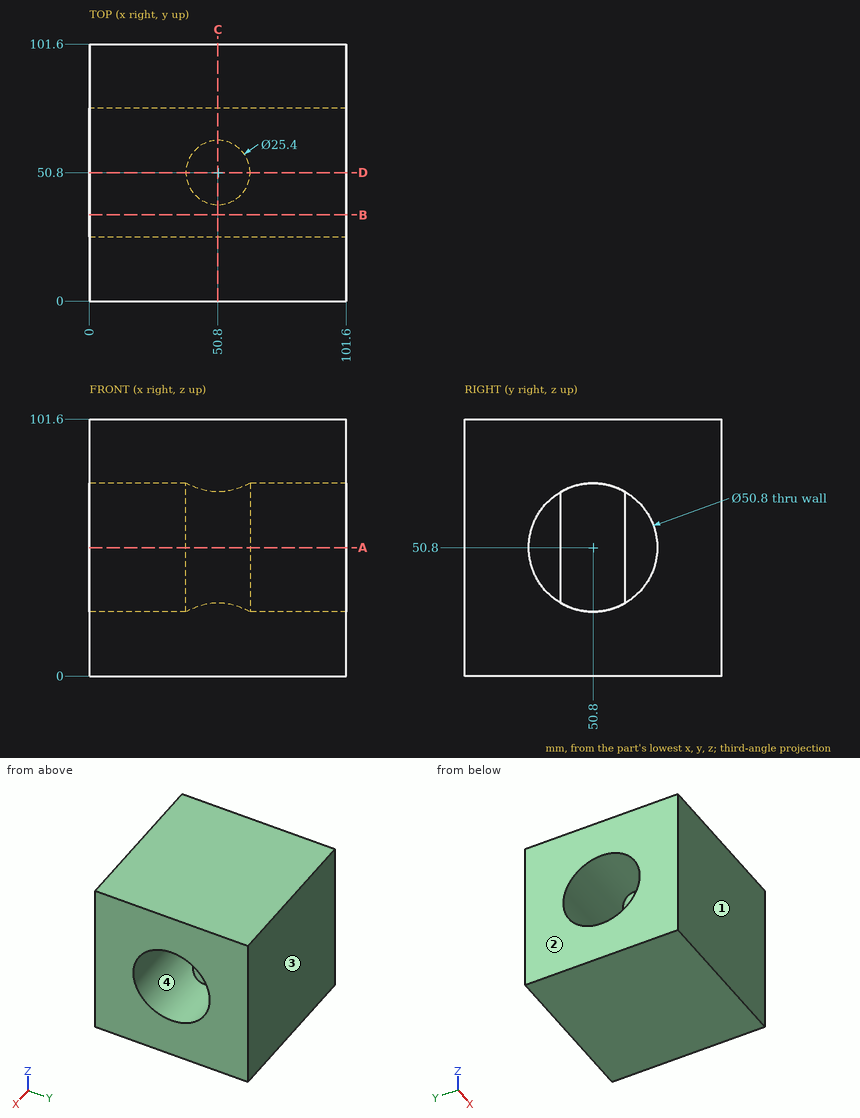
Input: dimensioned drawing with shaded views. Units: mm. Origin: part minimum x, y, z. Round coordinates to 2 decimals unless told otherwise and drop trailing zeros. Write each loop counter-clockwise with the first axis right and the second up, starting at its lowest first coordinate (ties: lowest second). Pieces come first, ordered by that corner, then holes. Notation, with made-up numbers: (32, -19) - (64, -19) arc R31 ccw to (64, 15) - close; hole circle Ø4 at (20, 58). An arc over 180 degrees is marked (long way). Write item = value, one per line.
(1) Pull-direction query (Y, two-part tool) for the marked faces 1, 2, 3 and 4; classes: +Y half, -Y half, draft (parallel to the pull), parting line (faces both ways), or undercut.
Geometry check:
face_1 = -Y half
face_2 = draft
face_3 = +Y half
face_4 = undercut
(2) Section query D-D on y = 50.8. Output: boundary loops of the cut face in (x, z).
Geometry check:
outline = (0, 0) - (101.6, 0) - (101.6, 25.4) - (63.5, 25.4) - (63.5, 76.2) - (101.6, 76.2) - (101.6, 101.6) - (0, 101.6) - (0, 76.2) - (38.1, 76.2) - (38.1, 25.4) - (0, 25.4) - close
(3) Section query A-A on z = 50.8. Output: boundary loops of the cut face in (x, y).
Geometry check:
outline = (0, 0) - (101.6, 0) - (101.6, 25.4) - (0, 25.4) - close; (0, 76.2) - (101.6, 76.2) - (101.6, 101.6) - (0, 101.6) - close; circle Ø25.4 at (50.8, 50.8)
(4) Section query C-C on x = 50.8. Output: boundary loops of the cut face in (y, z), then the cut area to 3 significant figures.
Geometry check:
outline = (0, 0) - (101.6, 0) - (101.6, 101.6) - (0, 101.6) - close; hole (38.1, 28.8) - (38.1, 72.8) arc R25.4 ccw to start; hole (63.5, 28.8) arc R25.4 ccw to (63.5, 72.8) - close
area = 9,530 mm^2
(5) Material intervals for probe 1 along Y at (x, z) = (55.5, 34.5); probe 2 along Z at (x, y) = (75, 50.8); probe 3 along Z at (x, y) = (78.5, 63), sorted ascending.
Geometry check:
probe_1 = 0 to 31.32, 39 to 62.6, 70.28 to 101.6
probe_2 = 0 to 25.4, 76.2 to 101.6
probe_3 = 0 to 28.52, 73.08 to 101.6
(6) Section query B-B on y = 34. Output: boundary loops of the cut face in (x, z).
Geometry check:
outline = (0, 0) - (101.6, 0) - (101.6, 31.75) - (0, 31.75) - close; (0, 69.85) - (101.6, 69.85) - (101.6, 101.6) - (0, 101.6) - close
